```python
from build123d import *

# Parameters (mm, degrees)
ESQUISSE1_W        = 24
ESQUISSE1_H        = 60
BOSS_EXTRU_1_DEPTH = 4
BOSS_EXTRU_2_DEPTH = 63


with BuildPart() as part:
    # Esquisse1 → Boss.-Extru.1 (new body)
    with BuildSketch(Plane.XY):
        with Locations((12, 30)):
            Rectangle(ESQUISSE1_W, ESQUISSE1_H)
    extrude(amount=BOSS_EXTRU_1_DEPTH)

    # Esquisse2 → Boss.-Extru.2 (add)
    with BuildSketch(Plane.XY.offset(4)):
        Polygon((24, 52.5), (20.3, 52.5), (20.3, 56.2), (4, 56.2), (4, 3.8), (20.3, 3.8), (20.3, 7.5), (24, 7.5), (24, 0), (0, 0), (0, 60), (24, 60), align=None)
    extrude(amount=BOSS_EXTRU_2_DEPTH)


solid = part.part
```
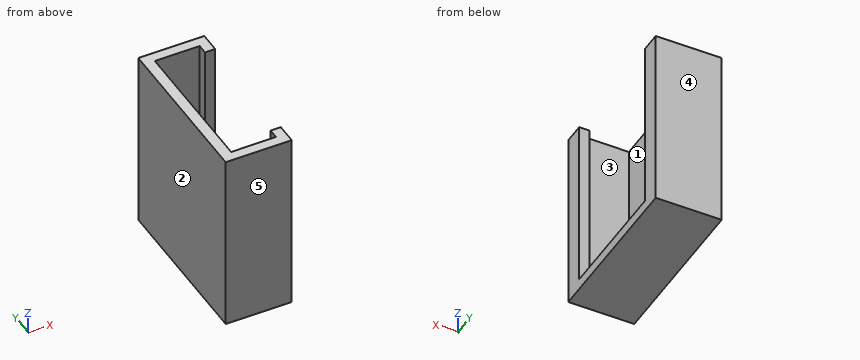
Check sheet for the modelled part. Datum: model origin and axes. Units: mm. Face numbers are marked on the shaded views. A direction names the side the tool comes from. Coordinates: 2 decimals unless noted, no trailing zeros. Loops run counter-clockwise (first coordinate to the right, second up) from the corner with the lowest first, then second, coordinate; pieces in that order, holes last.
1) Sectioned sample at D-D (y = 39). Record the boundary of the cut face in (x, z).
2) Material ranges on probe 1 along Y at (x, z) = (21.25, 21); probe 2 along Y at (x, z) = (16, 60); probe 3 along X at (y, z) = (53, 22), recorded low to high.
3) Gauge pin test, flat end, axial feed: pin 1 (5 mm diameter, centred on y = 31.5, z = 12.5, fed in from +X). Record the tip position at first contact, or that the pin passes through.
4) Sectioned sample at B-B (y = 5.5). Record the boundary of the cut face in (x, z), and give its area (3 significant figures).
5) Sectioned sample at C-C (z = 35). Record the boundary of the cut face in (x, y).
6) Release check for a two-part mould opening along Y. For the marked faces 3, 4 and 5 record: released by +Y, released by -Y, zero draft, split by the parting line, or undercut.
7) Sectioned sample at A-A (x = 9.75). Record the boundary of the cut face in (y, z), and give its area (3 significant figures).
8) Access from +Z, -Z, +X, -X, +Y, -Y to the whole of each face (thin tool, end or side, straight path). Record for the marked faces 1 and 2.
Check sheet entries:
1. outline: (0, 0) - (24, 0) - (24, 4) - (4, 4) - (4, 67) - (0, 67) - close
2. probe 1: y = 0 to 7.5, 52.5 to 60
2. probe 2: y = 0 to 3.8, 56.2 to 60
2. probe 3: x = 0 to 4, 20.3 to 24
3. pin 1: stops at x = 4
4. outline: (0, 0) - (24, 0) - (24, 67) - (20.3, 67) - (20.3, 4) - (4, 4) - (4, 67) - (0, 67) - close
4. area: 581 mm2
5. outline: (0, 0) - (24, 0) - (24, 7.5) - (20.3, 7.5) - (20.3, 3.8) - (4, 3.8) - (4, 56.2) - (20.3, 56.2) - (20.3, 52.5) - (24, 52.5) - (24, 60) - (0, 60) - close
6. face 3: undercut
6. face 4: released by +Y
6. face 5: released by -Y
7. outline: (0, 0) - (60, 0) - (60, 67) - (56.2, 67) - (56.2, 4) - (3.8, 4) - (3.8, 67) - (0, 67) - close
7. area: 719 mm2
8. face 1: +Z
8. face 2: +Z, -Z, -X, +Y, -Y
